from build123d import *

# Parameters (mm, degrees)
F1_DEPTH = 3.81
F4_DEPTH = 144.78
F5_SCALE = 0.5


with BuildPart() as f1:
    # F0 (on Front) → F1 (new body)
    with BuildSketch(Plane.XZ):
        Polygon((-37.1748663006, 21.2125933835), (-38.4448663006, 16.8945933835), (-33.8728663006, 16.8945933835), (-35.1428663006, 21.2125933835), align=None)
        Polygon((-33.8728663006, 16.8945933835), (-38.4448663006, 16.8945933835), (-38.4448663006, 12.5765933835), (106.3351336994, 12.5765933835), (106.3351336994, 16.8945933835), (101.7631336994, 16.8945933835), (100.2391336994, 16.8945933835), (95.6671336994, 16.8945933835), (94.1431336994, 16.8945933835), (89.5711336994, 16.8945933835), (88.0471336994, 16.8945933835), (83.4751336994, 16.8945933835), (81.9511336994, 16.8945933835), (77.3791336994, 16.8945933835), (75.8551336994, 16.8945933835), (71.2831336994, 16.8945933835), (69.7591336994, 16.8945933835), (65.1871336994, 16.8945933835), (63.6631336994, 16.8945933835), (59.0911336994, 16.8945933835), (57.5671336994, 16.8945933835), (52.9951336994, 16.8945933835), (51.4711336994, 16.8945933835), (46.8991336994, 16.8945933835), (45.3751336994, 16.8945933835), (40.8031336994, 16.8945933835), (39.2791336994, 16.8945933835), (34.7071336994, 16.8945933835), (33.1831336994, 16.8945933835), (28.6111336994, 16.8945933835), (27.0871336994, 16.8945933835), (22.5151336994, 16.8945933835), (20.9911336994, 16.8945933835), (16.4191336994, 16.8945933835), (14.8951336994, 16.8945933835), (10.3231336994, 16.8945933835), (8.7991336994, 16.8945933835), (4.2271336994, 16.8945933835), (2.7031336994, 16.8945933835), (-1.8688663006, 16.8945933835), (-3.3928663006, 16.8945933835), (-7.9648663006, 16.8945933835), (-9.4888663006, 16.8945933835), (-14.0608663006, 16.8945933835), (-15.5848663006, 16.8945933835), (-20.1568663006, 16.8945933835), (-21.6808663006, 16.8945933835), (-26.2528663006, 16.8945933835), (-27.7768663006, 16.8945933835), (-32.3488663006, 16.8945933835), align=None)
        Polygon((-31.0788663006, 21.2125933835), (-32.3488663006, 16.8945933835), (-27.7768663006, 16.8945933835), (-29.0468663006, 21.2125933835), align=None)
        Polygon((101.7631336994, 16.8945933835), (106.3351336994, 16.8945933835), (105.0651336994, 21.2125933835), (103.0331336994, 21.2125933835), align=None)
        Polygon((-24.9828663006, 21.2125933835), (-26.2528663006, 16.8945933835), (-21.6808663006, 16.8945933835), (-22.9508663006, 21.2125933835), align=None)
        Polygon((95.6671336994, 16.8945933835), (100.2391336994, 16.8945933835), (98.9691336994, 21.2125933835), (96.9371336994, 21.2125933835), align=None)
        Polygon((-18.8868663006, 21.2125933835), (-20.1568663006, 16.8945933835), (-15.5848663006, 16.8945933835), (-16.8548663006, 21.2125933835), align=None)
        Polygon((89.5711336994, 16.8945933835), (94.1431336994, 16.8945933835), (92.8731336994, 21.2125933835), (90.8411336994, 21.2125933835), align=None)
        Polygon((-12.7908663006, 21.2125933835), (-14.0608663006, 16.8945933835), (-9.4888663006, 16.8945933835), (-10.7588663006, 21.2125933835), align=None)
        Polygon((83.4751336994, 16.8945933835), (88.0471336994, 16.8945933835), (86.7771336994, 21.2125933835), (84.7451336994, 21.2125933835), align=None)
        Polygon((-6.6948663006, 21.2125933835), (-7.9648663006, 16.8945933835), (-3.3928663006, 16.8945933835), (-4.6628663006, 21.2125933835), align=None)
        Polygon((77.3791336994, 16.8945933835), (81.9511336994, 16.8945933835), (80.6811336994, 21.2125933835), (78.6491336994, 21.2125933835), align=None)
        Polygon((-0.5988663006, 21.2125933835), (-1.8688663006, 16.8945933835), (2.7031336994, 16.8945933835), (1.4331336994, 21.2125933835), align=None)
        Polygon((71.2831336994, 16.8945933835), (75.8551336994, 16.8945933835), (74.5851336994, 21.2125933835), (72.5531336994, 21.2125933835), align=None)
        Polygon((5.4971336994, 21.2125933835), (4.2271336994, 16.8945933835), (8.7991336994, 16.8945933835), (7.5291336994, 21.2125933835), align=None)
        Polygon((65.1871336994, 16.8945933835), (69.7591336994, 16.8945933835), (68.4891336994, 21.2125933835), (66.4571336994, 21.2125933835), align=None)
        Polygon((11.5931336994, 21.2125933835), (10.3231336994, 16.8945933835), (14.8951336994, 16.8945933835), (13.6251336994, 21.2125933835), align=None)
        Polygon((59.0911336994, 16.8945933835), (63.6631336994, 16.8945933835), (62.3931336994, 21.2125933835), (60.3611336994, 21.2125933835), align=None)
        Polygon((17.6891336994, 21.2125933835), (16.4191336994, 16.8945933835), (20.9911336994, 16.8945933835), (19.7211336994, 21.2125933835), align=None)
        Polygon((52.9951336994, 16.8945933835), (57.5671336994, 16.8945933835), (56.2971336994, 21.2125933835), (54.2651336994, 21.2125933835), align=None)
        Polygon((23.7851336994, 21.2125933835), (22.5151336994, 16.8945933835), (27.0871336994, 16.8945933835), (25.8171336994, 21.2125933835), align=None)
        Polygon((46.8991336994, 16.8945933835), (51.4711336994, 16.8945933835), (50.2011336994, 21.2125933835), (48.1691336994, 21.2125933835), align=None)
        Polygon((29.8811336994, 21.2125933835), (28.6111336994, 16.8945933835), (33.1831336994, 16.8945933835), (31.9131336994, 21.2125933835), align=None)
        Polygon((40.8031336994, 16.8945933835), (45.3751336994, 16.8945933835), (44.1051336994, 21.2125933835), (42.0731336994, 21.2125933835), align=None)
        Polygon((35.9771336994, 21.2125933835), (34.7071336994, 16.8945933835), (39.2791336994, 16.8945933835), (38.0091336994, 21.2125933835), align=None)
    extrude(amount=F1_DEPTH)

    # F3 (on plane+point) → F4 (join, through all)
    with BuildSketch(Plane.YZ.offset(106.3351336994)):
        Polygon((-11.43, 20.1965933835), (-11.43, 16.3865933835), (-11.43, 12.5765933835), (-3.81, 12.5765933835), (-3.81, 16.8945933835), (-7.62, 16.8945933835), (-7.62, 20.1965933835), align=None)
    extrude(amount=-F4_DEPTH)


with BuildPart() as f1_1:
    # F5: moved
    add(f1.part.scale(F5_SCALE).moved(Location((-19.2224331503, 0, 6.2882966917))))


solid = f1_1.part
Could you check a few things on this model? Use its own coordinates, in mm. A direction names the side the tool comes from. Give positions to 0.01 mm unless a question says otherwise; leave off trailing zeros.
1. Suppose I cut it at A-A (z = 15.4). Give the number of separate pieces and of enclosed holes in the cut face, plus the area to 3 significant figures.
2. For faces 1 (the flat face through (-28, -1.905, 16)), 2 (the flat face through (7.597, -0.939, 15.83)), which set-ups out of +Z, -Z, +X, -X, +Y, -Y let a thin tool reach every point of the face, with its end or its side?
3. I need wall thicknesses on L1, parallel to Y at x = -32, z = 15.05 (3 decimals); L2, parallel to Z at x = 26, y = -3.4; L3, parallel to Z at x = 6, y = -4.75. Which ranges of each line are inside material? Lowest first, please.
4. Will this pin go through, and if not, where does the flat tip stop? P1, Ø0.6, axis at x = -14.5, y = -5, coming from the +Z side.
5. We'd pull the mould along X, two halves only. Please class faces 3 (the flat face through (-25.93, -0.94, 15.83)), 4 (the flat face through (27, -1.905, 16)): pulls with the +X half, pulls with the -X half, needs draft (parallel to the pull), parting line crosses it, or undercut.
Solved:
1. separate pieces: 25
1. enclosed holes: 0
1. area: 225 mm2
2. face 1: +Z, +X, -X
2. face 2: +Z, +Y
3. L1: y = -5.715 to -3.81, -1.905 to 0
3. L2: z = 12.58 to 14.74
3. L3: z = 12.58 to 16.39
4. P1: stops at z = 16.39
5. face 3: undercut
5. face 4: needs draft
